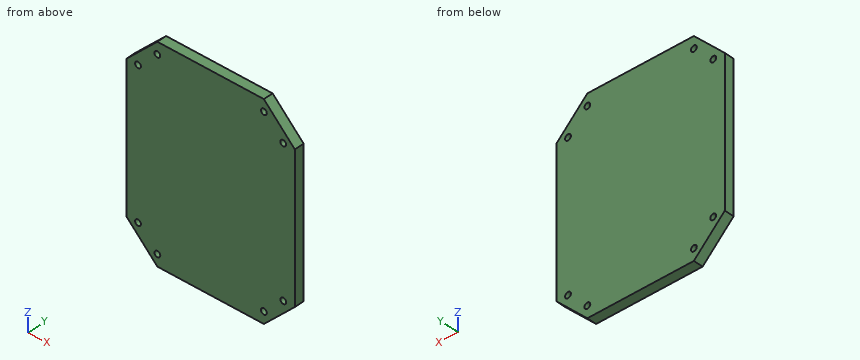
from build123d import *

# Parameters (mm, degrees)
BOSS_EXTRUDE1_DEPTH          = 5
F_3_0_3_DIAMETER_HOLE2_D     = 3
F_3_0_3_DIAMETER_HOLE2_DEPTH = 5
F_3_0_3_DIAMETER_HOLE3_D     = 3
F_3_0_3_DIAMETER_HOLE3_DEPTH = 5
F_3_0_3_DIAMETER_HOLE4_D     = 3
F_3_0_3_DIAMETER_HOLE4_DEPTH = 5


with BuildPart() as part:
    # Sketch1 → Boss-Extrude1 (new body)
    with BuildSketch(Plane(origin=(0, 0, 0), x_dir=(1, 0, 0), z_dir=(0, 1, 0))):
        Polygon((-36.833168475, 10.918963515), (-20.85333758, 26.89879441), (34.14666242, 26.89879441), (50.126493315, 10.918963515), (50.126493315, -64.081036485), (34.14666242, -80.060867381), (-20.85333758, -80.060867381), (-36.833168475, -64.081036485), align=None)
    extrude(amount=BOSS_EXTRUDE1_DEPTH)

    # Ø3.0 (3) Diameter Hole2
    with Locations(Plane(origin=(-30.85333758, 5, -10.918963515), x_dir=(0, 0, 1), z_dir=(0, 1, 0))):
        with Locations((0, 0), (-10, 10)):
            Hole(F_3_0_3_DIAMETER_HOLE2_D / 2, depth=F_3_0_3_DIAMETER_HOLE2_DEPTH)

    # Ø3.0 (3) Diameter Hole3
    with Locations(Plane(origin=(34.14666242, 5, -20.918963515), x_dir=(0, 0, 1), z_dir=(0, 1, 0))):
        with Locations((0, 0), (10, 10)):
            Hole(F_3_0_3_DIAMETER_HOLE3_D / 2, depth=F_3_0_3_DIAMETER_HOLE3_DEPTH)

    # Ø3.0 (3) Diameter Hole4
    with Locations(Plane(origin=(-30.85333758, 5, 64.081036485), x_dir=(0, 0, 1), z_dir=(0, 1, 0))):
        with Locations((0, 0), (10, 10), (10, 65), (0, 75)):
            Hole(F_3_0_3_DIAMETER_HOLE4_D / 2, depth=F_3_0_3_DIAMETER_HOLE4_DEPTH)


solid = part.part
CAD build for the part. Positions are in the model's coordinates, mm. Round coordinates to 2 decimals unless told otherwise and drop trailing zeros. Write each loop counter-clockwise with the first axis right and the second up, starting at its lowest first coordinate (ties: lowest second). Pieces come first, ordered by that corner, then holes.
(1) Probe line 1 along Z through (x, y) = (43, 2.85); line 2 along X through (y, z) = (1.4, 63); line 3 along X through (y, z) = (1.5, -21). List the from-to ranges inside material, lowest first.
(2) Slice it at A-A, the plane y = 2.95. Count the separate pieces of the cut face and the enclosed holes in it, and give its area (3 significant figures).
(3) Drop a flat-ended pin along its axis: P1, Ø2.5, axis at x = 44.15, z = 64.08, coming from the -Y side. Give the stop position or say it passes through.
(4) Slice it at B-B, the plane x = -24. Write the cut outline in (y, z).
(5) Slice it at C-C, the plane z = 67. Write the cut outline in (x, y), and give its area (3 significant figures).
From the geometry:
1. line 1: z = -18.05 to -11.89, -9.95 to 63.11, 65.05 to 71.21
1. line 2: x = -36.83 to -31.89, -29.81 to 43.11, 45.19 to 50.13
1. line 3: x = -26.75 to -22.35, -19.36 to 32.65, 35.64 to 40.05
2. separate pieces: 1
2. enclosed holes: 8
2. area: 8,730 mm2
3. P1: passes through
4. outline: (0, -23.75) - (5, -23.75) - (5, 76.91) - (0, 76.91) - close
5. outline: (-33.91, 0) - (47.21, 0) - (47.21, 5) - (-33.91, 5) - close
5. area: 406 mm2
